Can you work these out from the model? Positions are in its coordinate system, mm. A direction names the side the tool comes from. Give positions to 0.01 mm unless a question says otherwise; leave off trailing zeros. Write each loop counter-clockwise with the first axis right and the second up, starting at its lowest first coordinate (ties: lowest second). Pieces come first, ordered by that corner, then holes.
1. If I drill on probe 1 along X at (y, z) = (74.65, 25.4); probe 2 along Z at (x, y) = (-51, 38.1); probe 3 along Z at (x, y) = (-50.8, 29), over which ranges is the centre line in solid material (lowest first)?
2. I'm going to push flat-ended pins straight in: pin 1 (9 mm diameter, centred on x = 51, z = -27, fed in from +Y); pin 2 (10 mm diameter, centred on x = 50.8, z = -25.4, fed in from +Y); pin 3 (5 mm diameter, centred on x = -50.8, z = 25.4, fed in from -Y); pin 4 (9 mm diameter, centred on x = 52, z = 26, fed in from +Y). Where does each tip first touch, or does it pass through?
3. Thinking about a two-plate mould opening in X: for faces 3 (the flat face through (-1, 0, -1)), 4 (the cylindrical face through (48.433, 37.049, 26.909)), which applies, pulls with the +X half, pulls with the -X half, needs draft (parallel to the pull), parting line crosses it, or undercut?
4. Suppose I cut it at B-B (y = 38.1). Please give me the cut outline in (x, z).
5. On a 3-axis mill with a long thin cutter (end or side, diameter ignored), from which of +Z, -Z, +X, -X, +Y, -Y can I reach the whole of each face in a straight line? I mean faces 1 (the flat face through (-1, 76.2, 11)), 2 (the cylindrical face through (-54.555, 74.338, -29.495)). Say none if no direction works.
6. Suppose I cut it at A-A (z = -25.4). Please give me the cut outline in (x, y) (3 decimals), and give its area (3 significant figures).
7. Suppose I cut it at C-C (x = -50.8). Please give me the cut outline in (y, z) (3 decimals).
```python
from build123d import *

# Parameters (mm, degrees)
SKETCH1_W                                       = 152.4
SKETCH1_H                                       = 101.6
BOSS_EXTRUDE1_DEPTH                             = 76.2
CBORE_FOR_10_BINDING_HEAD_MACHINE_S_2_COUNT     = 2
CBORE_FOR_10_BINDING_HEAD_MACHINE_S_2_PITCH     = 101.6
CBORE_FOR_10_BINDING_HEAD_MACHINE_S_3_COUNT     = 2
CBORE_FOR_10_BINDING_HEAD_MACHINE_S_3_PITCH     = 113.592253257
CBORE_FOR_10_BINDING_HEAD_MACHINE_S_4_COUNT     = 2
CBORE_FOR_10_BINDING_HEAD_MACHINE_S_4_PITCH     = 50.8
CSK_FOR_M6_FLAT_HEAD_MACHINE_SCREW1_D           = 6.4
CSK_FOR_M6_FLAT_HEAD_MACHINE_SCREW1_DEPTH       = 50.8
CSK_FOR_M6_FLAT_HEAD_MACHINE_SCREW1_CSINK_D     = 12.6
CSK_FOR_M6_FLAT_HEAD_MACHINE_SCREW1_CSINK_ANGLE = 100
CSK_FOR_M6_FLAT_HEAD_MACHINE_SCREW1_TIP         = 1.922753981
F_7_16_14_TAPPED_HOLE1_D                        = 9.3472
F_7_16_14_TAPPED_HOLE1_ON_FACE_2_D              = 9.3472


with BuildPart() as part:
    # Sketch1 → Boss-Extrude1 (new body)
    with BuildSketch(Plane(origin=(0, 0, 0), x_dir=(1, 0, 0), z_dir=(0, 1, 0))):
        Rectangle(SKETCH1_W, SKETCH1_H)
    extrude(amount=BOSS_EXTRUDE1_DEPTH)

    # Sketch7 → CBORE for #10 Binding Head Machine Screw2 (revolve, cut)
    with BuildSketch(Plane(origin=(-50.8, 76.2, -25.4), x_dir=(0, 0, 1), z_dir=(1, 0, 0))):
        Polygon((0, 0), (0, 76.2), (2.8067, 76.2), (2.8067, 3.1242), (5.55625, 3.1242), (5.55625, 0.635), (6.19125, 0), align=None)
    cbore_for_10_binding_head_machine_screw = revolve(axis=Axis((-50.8, 82.55, -25.4), (0, -1, 0)), mode=Mode.SUBTRACT)

    # CBORE for _10 Binding Head Machine S 2: CBORE for #10 Binding Head Machine Screw2 ×2
    with Locations(*[(i * CBORE_FOR_10_BINDING_HEAD_MACHINE_S_2_PITCH, 0, 0) for i in range(1, CBORE_FOR_10_BINDING_HEAD_MACHINE_S_2_COUNT)]):
        add(cbore_for_10_binding_head_machine_screw, mode=Mode.SUBTRACT)

    # CBORE for _10 Binding Head Machine S 3: CBORE for #10 Binding Head Machine Screw2 ×2
    with Locations(*[Vector(0.894427191, 0, 0.447213595) * (i * CBORE_FOR_10_BINDING_HEAD_MACHINE_S_3_PITCH) for i in range(1, CBORE_FOR_10_BINDING_HEAD_MACHINE_S_3_COUNT)]):
        add(cbore_for_10_binding_head_machine_screw, mode=Mode.SUBTRACT)

    # CBORE for _10 Binding Head Machine S 4: CBORE for #10 Binding Head Machine Screw2 ×2
    with Locations(*[(0, 0, i * CBORE_FOR_10_BINDING_HEAD_MACHINE_S_4_PITCH) for i in range(1, CBORE_FOR_10_BINDING_HEAD_MACHINE_S_4_COUNT)]):
        add(cbore_for_10_binding_head_machine_screw, mode=Mode.SUBTRACT)

    # CSK for M6 Flat Head Machine Screw1
    with Locations(Plane(origin=(0, 76.2, 0), x_dir=(1, 0, 0), z_dir=(0, 1, 0))):
        with Locations((0, 0)):
            CounterSinkHole(CSK_FOR_M6_FLAT_HEAD_MACHINE_SCREW1_D / 2, CSK_FOR_M6_FLAT_HEAD_MACHINE_SCREW1_CSINK_D / 2, depth=CSK_FOR_M6_FLAT_HEAD_MACHINE_SCREW1_DEPTH, counter_sink_angle=CSK_FOR_M6_FLAT_HEAD_MACHINE_SCREW1_CSINK_ANGLE)
            with Locations((0, 0, -(CSK_FOR_M6_FLAT_HEAD_MACHINE_SCREW1_DEPTH + CSK_FOR_M6_FLAT_HEAD_MACHINE_SCREW1_TIP / 2))):  # 118° drill point
                Cone(0, CSK_FOR_M6_FLAT_HEAD_MACHINE_SCREW1_D / 2, CSK_FOR_M6_FLAT_HEAD_MACHINE_SCREW1_TIP, mode=Mode.SUBTRACT)

    # 7/16-14 Tapped Hole1 (through all)
    with Locations(Plane(origin=(0, 38.1, 50.8), x_dir=(1, 0, 0), z_dir=(0, 0, 1))):
        with Locations((0, 0)):
            Hole(F_7_16_14_TAPPED_HOLE1_D / 2)

    # 7/16-14 Tapped Hole1 on face 2 (through all)
    with Locations(Plane(origin=(76.2, 38.1, 0), x_dir=(0, 0, 1), z_dir=(1, 0, 0))):
        with Locations((0, 0)):
            Hole(F_7_16_14_TAPPED_HOLE1_ON_FACE_2_D / 2)


solid = part.part
```
Checks:
1. probe 1: x = -76.2 to -56.36, -45.24 to 45.24, 56.36 to 76.2
1. probe 2: z = -50.8 to -28.2, -22.6 to -4.67, 4.67 to 22.6, 28.2 to 50.8
1. probe 3: z = -50.8 to -28.21, -22.59 to 22.59, 28.21 to 50.8
2. pin 1: stops at y = 76.12
2. pin 2: stops at y = 73.08
2. pin 3: passes through
2. pin 4: stops at y = 75.85
3. face 3: needs draft
3. face 4: undercut
4. outline: (-76.2, -50.8) - (-4.67, -50.8) - (-4.67, -4.67) - (-76.2, -4.67) - close; (-76.2, 4.67) - (-4.67, 4.67) - (-4.67, 50.8) - (-76.2, 50.8) - close; (4.67, -50.8) - (76.2, -50.8) - (76.2, -4.67) - (4.67, -4.67) - close; (4.67, 4.67) - (76.2, 4.67) - (76.2, 50.8) - (4.67, 50.8) - close; hole circle Ø5.61 at (-50.8, -25.4); hole circle Ø5.61 at (-50.8, 25.4); hole circle Ø5.61 at (50.8, -25.4); hole circle Ø5.61 at (50.8, 25.4)
5. face 1: +Z, -Z, +X, -X, +Y
5. face 2: +Y
6. outline: (-76.2, 0) - (-53.607, 0) - (-53.607, 73.076) - (-56.356, 73.076) - (-56.356, 75.565) - (-56.991, 76.2) - (-76.2, 76.2) - close; (-47.993, 0) - (47.993, 0) - (47.993, 73.076) - (45.244, 73.076) - (45.244, 75.565) - (44.609, 76.2) - (-44.609, 76.2) - (-45.244, 75.565) - (-45.244, 73.076) - (-47.993, 73.076) - close; (53.607, 0) - (76.2, 0) - (76.2, 76.2) - (56.991, 76.2) - (56.356, 75.565) - (56.356, 73.076) - (53.607, 73.076) - close; hole circle Ø9.347 at (0, 38.1)
6. area: 10,700 mm2
7. outline: (0, -50.8) - (76.2, -50.8) - (76.2, -31.591) - (75.565, -30.956) - (73.076, -30.956) - (73.076, -28.207) - (0, -28.207) - close; (0, -22.593) - (73.076, -22.593) - (73.076, -19.844) - (75.565, -19.844) - (76.2, -19.209) - (76.2, 19.209) - (75.565, 19.844) - (73.076, 19.844) - (73.076, 22.593) - (0, 22.593) - close; (0, 28.207) - (73.076, 28.207) - (73.076, 30.956) - (75.565, 30.956) - (76.2, 31.591) - (76.2, 50.8) - (0, 50.8) - close; hole circle Ø9.347 at (38.1, 0)
